from build123d import *

# Parameters (mm, degrees)
ESQUISSE1_W             = 5
ESQUISSE1_H             = 20.2
BOSS_EXTRU_1_DEPTH      = 13.9
ESQUISSE4_R             = 1.05
ENL_V_MAT_EXTRU_1_DEPTH = 18.362891464
SKETCH1_R               = 3
BOSS_EXTRUDE1_DEPTH     = 1


with BuildPart() as part:
    # Esquisse1 → Boss.-Extru.1 (new body)
    with BuildSketch(Plane.XY):
        Rectangle(ESQUISSE1_W, ESQUISSE1_H)
    extrude(amount=BOSS_EXTRU_1_DEPTH)

    # Esquisse4 → Enlèv. mat.-Extru.1 (cut, through all)
    with BuildSketch(Plane(origin=(0, 0, 0), x_dir=(-1, 0, 0), z_dir=(0, 0, -1))):
        with Locations((0, 5)):
            Circle(ESQUISSE4_R)
        with Locations((0, -5)):
            Circle(ESQUISSE4_R)
    extrude(amount=-ENL_V_MAT_EXTRU_1_DEPTH, mode=Mode.SUBTRACT)

    # Sketch1 → Boss-Extrude1 (add)
    with BuildSketch(Plane.ZY.offset(2.5)):
        with Locations(Location((6.95, 0, 0), (0, 0, 270))):
            Circle(SKETCH1_R)
    extrude(amount=BOSS_EXTRUDE1_DEPTH)

    # Sketch5 → Revolve4 (revolve)
    with BuildSketch(Plane(origin=(0, 0, 0), x_dir=(-1, 0, 0), z_dir=(0, -1, 0))):
        with BuildLine():
            Line((3.5, -6.95), (12.5, -6.95))
            ThreePointArc((12.5, -6.95), (9.08113883, -11.69341649), (3.5, -9.95))
            Line((3.5, -9.95), (3.5, -6.95))
        make_face()
    revolve(axis=Axis((-3.5, 0, 6.95), (-1, 0, 0)))


solid = part.part
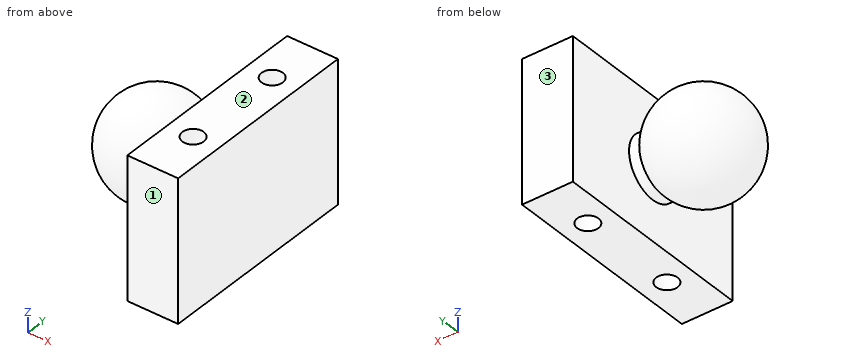
Geometry: final body of the model. Coordinates: model frame, mm. Face numbers are marked on the shaded views. Give positions to 0.01 mm unless a question says otherwise; leave off trailing zeros. Loops run counter-clockwise (first coordinate to the right, second up) from the corner with the lowest first, then second, coordinate; pieces in that order, holes last. Notation, with made-up numbers: (32.5, -18.5) - (61.5, -18.5) arc R20 cw to (61.5, 10.5) - close; hole circle Ø2 at (83, 73). An arc over 180 degrees is marked (long way). One line per question, with ' | ' between items. Start each with the question number.
(1) Section query A-A on x = 0. Return loops of the section in (y, z).
(2) Pull-direction query (Y, two-part tool) for the marked faces 1, 2 and 3; classes: released by +Y, released by -Y, zero draft, split by the parting line, or undercut.
(3) Section query D-D on z = 6.95. Return loops of the section in (x, y), then the cut area to 3 significant figures.
(4) Contact query for flat-ended pins moving along their axis: pin 1 (1.9 mm diameter, centred on x = 0, y = -5, fed in from -Z); pin 2 (1.5 mm diameter, centred on y = 6.5, z = 3, fed in from -X); pin 3 (2 mm diameter, centred on x = -4.5, z = 4.5, fed in from +Y); pin 4 (3 mm diameter, centred on x = -7.5, z = 9.5, fed in from -Y). Output: stop coordinate, or through.
(5) Ray query, line 1 (Y direction, x = 0, z = 10.5); line 2 (Y direction, x = 0.5, z = 7.25); line 3 (X direction, y = 9, z = 13.25). Return the intervals inside material, ascending. Write a range as from..to.
(6) Section query C-C on y = -4.5. Return loops of the section in (x, z).
(7) Section query B-B on z = 10.25. Return loops of the section in (x, y), then the cut area to 3 significant figures.
The answers:
1) outline: (-10.1, 0) - (-6.05, 0) - (-6.05, 13.9) - (-10.1, 13.9) - close; (-3.95, 0) - (3.95, 0) - (3.95, 13.9) - (-3.95, 13.9) - close; (6.05, 0) - (10.1, 0) - (10.1, 13.9) - (6.05, 13.9) - close
2) face 1: released by -Y | face 2: zero draft | face 3: released by +Y
3) outline: (-3.5, -3) - (-2.5, -3) - (-2.5, -10.1) - (2.5, -10.1) - (2.5, 10.1) - (-2.5, 10.1) - (-2.5, 3) - (-3.5, 3) arc R5 ccw (long way) to start; hole circle Ø2.1 at (0, -5); hole circle Ø2.1 at (0, 5) | area: 175 mm2
4) pin 1: through | pin 2: x = -2.5 | pin 3: y = 4.09 | pin 4: y = -4.89
5) line 1: -10.1..-6.05, -3.95..3.95, 6.05..10.1 | line 2: -10.1..-5.92, -4.08..4.08, 5.92..10.1 | line 3: -2.5..2.5
6) outline: circle Ø4.36 at (-7.5, 6.95); (-2.5, 0) - (-0.92, 0) - (-0.92, 13.9) - (-2.5, 13.9) - close; (0.92, 0) - (2.5, 0) - (2.5, 13.9) - (0.92, 13.9) - close
7) outline: circle Ø7.51 at (-7.5, 0); (-2.5, -10.1) - (2.5, -10.1) - (2.5, 10.1) - (-2.5, 10.1) - close; hole circle Ø2.1 at (0, -5); hole circle Ø2.1 at (0, 5) | area: 138 mm2
